Can you work these out from the model? Positions are in its coordinate system, mm. Face numbers are marked on the shaded views. Give positions to 0.01 mm unless a question says otherwise; leave off trailing zeros. Loops run counter-clockwise (first coordinate to the right, second up) from the corner with the lowest first, then second, coordinate; pieces in that order, holes last. Notation, with made-up numbers: (82.5, 55.5) - (139.5, 55.5) arc R19 ccw to (139.5, 65.5) - close; hole circle Ø4 at (53.5, 1). An arc over 180 degrees is marked (long way). Answer as a JSON object with one key per item and string values.
```python
from build123d import *

# Parameters (mm, degrees)
SKETCH1_R             = 27.55
SKETCH1_R_2           = 11
BOSS_EXTRUDE1_DEPTH   = 3
SKETCH1_3_R           = 31.55
SKETCH1_3_R_2         = 27.55
BOSS_EXTRUDE2_DEPTH   = 2
M3X0_5_TAPPED_HOLE1_D = 2.5
SKETCH6_R             = 3.5
SKETCH6_R_2           = 2.5
CUT_EXTRUDE1_DEPTH    = 45.719179331
CIRPATTERN1_COUNT     = 6


with BuildPart() as part:
    # Sketch1 → Boss-Extrude1 (new body)
    with BuildSketch(Plane(origin=(0, 0, 0), x_dir=(1, 0, 0), z_dir=(0, 1, 0))):
        with Locations(Location((0, 0, 0), (0, 0, 270))):
            Circle(SKETCH1_R)
        with Locations(Location((0, 0, 0), (0, 0, 270))):
            Circle(SKETCH1_R_2, mode=Mode.SUBTRACT)
    extrude(amount=BOSS_EXTRUDE1_DEPTH)

    # Sketch1_3 → Boss-Extrude2 (add)
    with BuildSketch(Plane(origin=(0, 0, 0), x_dir=(1, 0, 0), z_dir=(0, 1, 0))):
        with Locations(Location((0, 0, 0), (0, 0, 270))):
            Circle(SKETCH1_3_R)
        with Locations(Location((0, 0, 0), (0, 0, 270))):
            Circle(SKETCH1_3_R_2, mode=Mode.SUBTRACT)
    extrude(amount=BOSS_EXTRUDE2_DEPTH)

    # M3x0.5 Tapped Hole1 (through all)
    with Locations(Plane(origin=(0, 3, 0), x_dir=(1, 0, 0), z_dir=(0, 1, 0))):
        with Locations((0, 15)):
            m3x0_5_tapped_hole1 = Hole(M3X0_5_TAPPED_HOLE1_D / 2)

    # Sketch6 → Cut-Extrude1 (cut, through all)
    with BuildSketch(Plane(origin=(0, 3, 0), x_dir=(1, 0, 0), z_dir=(0, 1, 0))):
        with Locations(Location((20, 0, 0), (0, 0, 270))):
            Circle(SKETCH6_R)
        with Locations(Location((0, 23, 0), (0, 0, 270))):
            Circle(SKETCH6_R_2)
    cut_extrude1 = extrude(amount=-CUT_EXTRUDE1_DEPTH, mode=Mode.SUBTRACT)

    # CirPattern1: M3x0.5 Tapped Hole1, Cut-Extrude1 ×6 about axis
    cirpattern1_axis = Axis((0, 0, 0), (0, 1, 0))
    add([m3x0_5_tapped_hole1.rotate(cirpattern1_axis, i * 360 / CIRPATTERN1_COUNT) for i in range(1, CIRPATTERN1_COUNT)], mode=Mode.SUBTRACT)
    add([cut_extrude1.rotate(cirpattern1_axis, i * 360 / CIRPATTERN1_COUNT) for i in range(1, CIRPATTERN1_COUNT)], mode=Mode.SUBTRACT)


solid = part.part
```
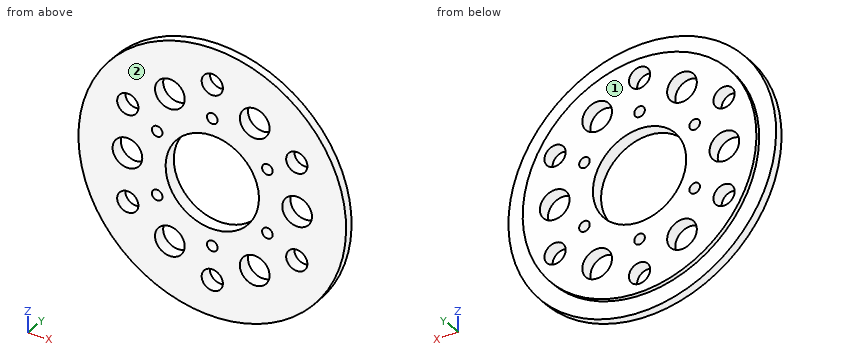
1) I'm going to push flat-ended pins straight in: P1, Ø19, axis at x = 8, z = 6.5, coming from the +Y side; P2, Ø1, axis at x = 22, y = 1, coming from the +Z side; P3, Ø3, axis at x = 20.5, z = 23, coming from the +Y side. Where does each tip first touch, or does it pass through?
Check sheet entries:
{"P1": "y = 3", "P2": "z = 23.09", "P3": "y = 2"}
2) I need wall thicknesses on L1, parallel to X at y = 2.55, z = -3; L2, parallel to Z at x = 18.5, y = 0.5; L3, parallel to Z at x = 14, y = 1.9. Which ranges of each line are inside material? Lowest first, please.
Check sheet entries:
{"L1": "-27.39 to -21.8, -18.2 to -10.58, 10.58 to 18.2, 21.8 to 27.39", "L2": "-25.56 to -13.56, -9.44 to -3.16, 3.16 to 9.44, 13.56 to 25.56", "L3": "-28.27 to -8.24, -6.76 to 6.76, 8.24 to 28.27"}
3) Imagine slicing it at C-C on x = 10. Write out the boundary of the cut face in (y, z).
Check sheet entries:
{"outline": "(0, -29.92) - (2, -29.92) - (2, -25.67) - (3, -25.67) - (3, -20.82) - (0, -20.82) - close; (0, -13.82) - (3, -13.82) - (3, -4.58) - (0, -4.58) - close; (0, 4.58) - (3, 4.58) - (3, 13.82) - (0, 13.82) - close; (0, 20.82) - (3, 20.82) - (3, 25.67) - (2, 25.67) - (2, 29.92) - (0, 29.92) - close"}
4) Imagine slicing it at D-D on y = 1.3. Give the number of separate pieces and of enclosed holes in the cut face, and give its area (3 significant figures).
Check sheet entries:
{"separate pieces": "1", "enclosed holes": "19", "area": "2,370 mm2"}
5) Imagine slicing it at B-B on z = -7.5. Write out the boundary of the cut face in (x, y), and give its area (3 significant figures).
Check sheet entries:
{"outline": "(-30.65, 0) - (-14.24, 0) - (-14.24, 3) - (-26.51, 3) - (-26.51, 2) - (-30.65, 2) - close; (-11.74, 0) - (-8.05, 0) - (-8.05, 3) - (-11.74, 3) - close; (8.05, 0) - (11.74, 0) - (11.74, 3) - (8.05, 3) - close; (14.24, 0) - (30.65, 0) - (30.65, 2) - (26.51, 2) - (26.51, 3) - (14.24, 3) - close", "area": "112 mm2"}
6) If we mould it in two halves opening along Y, with no side actions, what happens to the marked faces 1 and 2? For each: released by +Y, released by -Y, zero draft, split by the parting line, or undercut.
Check sheet entries:
{"face 1": "released by +Y", "face 2": "released by -Y"}
7) Imagine slicing it at A-A on x = 0. Write out the boundary of the cut face in (y, z), and give its area (3 significant figures).
Check sheet entries:
{"outline": "(0, -31.55) - (2, -31.55) - (2, -27.55) - (3, -27.55) - (3, -25.5) - (0, -25.5) - close; (0, -20.5) - (3, -20.5) - (3, -16.25) - (0, -16.25) - close; (0, -13.75) - (3, -13.75) - (3, -11) - (0, -11) - close; (0, 11) - (3, 11) - (3, 13.75) - (0, 13.75) - close; (0, 16.25) - (3, 16.25) - (3, 20.5) - (0, 20.5) - close; (0, 25.5) - (3, 25.5) - (3, 27.55) - (2, 27.55) - (2, 31.55) - (0, 31.55) - close", "area": "70.3 mm2"}
